For this review, take the finished solid that the model builds, in its own axes (mm). Give positions to 0.01 mm unless a question says otherwise; leave off trailing zeros. Loops run counter-clockwise (first coordinate to the right, second up) from the corner with the lowest first, then second, coordinate; pieces in that order, holes last.
```python
from build123d import *

# Parameters (mm, degrees)
SKETCH1_R           = 3.3782
BOSS_EXTRUDE1_DEPTH = 3.175
FILLET1_R           = 25.4


with BuildPart() as part:
    # Sketch1 → Boss-Extrude1 (new, symmetric)
    with BuildSketch(Plane(origin=(-76.913317281, 0, 0), x_dir=(0, 0, -1), z_dir=(1, 0, 0))):
        with BuildLine():
            Line((535.218804975, 907.961983625), (418.2911251, 916.04381761))
            Line((418.2911251, 916.04381761), (190.115926381, 1052.658490892))
            Line((190.115926381, 1052.658490892), (172.155048622, 1087.522632949))
            ThreePointArc((172.155048622, 1087.522632949), (173.529973777, 1095.130662847), (181.234623159, 1095.771690164))
            Line((181.234623159, 1095.771690164), (418.2911251, 943.327259155))
            Line((418.2911251, 943.327259155), (537.059525989, 923.712003677))
            ThreePointArc((537.059525989, 923.712003677), (543.649965664, 914.959198723), (535.218804975, 907.961983625))
        make_face()
        with Locations((177.8, 1090.430729224)):
            Circle(SKETCH1_R, mode=Mode.SUBTRACT)
        with Locations((434.1661251, 925.56881761)):
            Circle(SKETCH1_R, mode=Mode.SUBTRACT)
        with Locations((535.7661251, 915.880591264)):
            Circle(SKETCH1_R, mode=Mode.SUBTRACT)
    extrude(amount=BOSS_EXTRUDE1_DEPTH, both=True)

    # Fillet1
    fillet1_edges = [part.edges().sort_by_distance(p)[0] for p in [
        (-76.913317281, 916.04381761, -418.2911251),
        (-76.913317281, 1052.658490892, -190.115926381),
        (-76.913317281, 943.327259155, -418.2911251),
    ]]
    fillet(fillet1_edges, radius=FILLET1_R)


solid = part.part
```
Q1. Consider section B-B on x = -78.25. Count the separate pieces of the cut face and the enclosed holes in it, plus the area to 3 significant figures.
Answers:
separate pieces: 1
enclosed holes: 3
area: 10,300 mm2
Q2. Consider section A-A on z = -177.8. Give the boundary of the cut face in (x, y).
Answers:
outline: (-80.09, 1076.57) - (-73.74, 1076.57) - (-73.74, 1087.05) - (-80.09, 1087.05) - close; (-80.09, 1093.81) - (-73.74, 1093.81) - (-73.74, 1096.78) - (-80.09, 1096.78) - close
Q3. Consider section C-C on z = -455. Give the boundary of the cut face in (x, y).
Answers:
outline: (-80.09, 913.51) - (-73.74, 913.51) - (-73.74, 937.26) - (-80.09, 937.26) - close
Q4. Mouldability with a two-part tool opening along Y and no side actions: class faces 1 (the flat face through (-73.738, 982, -345)), 2 (the flat face through (-76.87, 911.74, -480.57)), 3 (the cylindrical face through (-76.958, 1087.133, -177.068)) as +Y half, -Y half, draft (parallel to the pull), parting line (faces both ways), or undercut.
Answers:
face 1: draft
face 2: -Y half
face 3: undercut
Q5. For pin 1 Ø4 at (y, z) = (1090.43, -177.8) entering from -X; pin 2 Ø2 at (x, z) = (-74.5, -285.5) entering from +Y; pin 3 Ø1 at (x, z) = (-75, -311) entering from -Y, all flat-tipped, find the tip position at first contact; note any pin that passes through.
Answers:
pin 1: passes through
pin 2: stops at y = 1029.36
pin 3: stops at y = 979.98
Q6. Consider section D-D on y = 1066.5. Give the boundary of the cut face in (x, z).
Answers:
outline: (-80.09, -226.75) - (-73.74, -226.75) - (-73.74, -182.99) - (-80.09, -182.99) - close
Q7. For probe 1 along Y at (x, z) = (-77, -177.8); probe 2 along Z at (x, y) = (-75, 951); probe 3 along Z at (x, y) = (-79.5, 967), list the stretches that pass through material, from the lowest coordinate up.
Answers:
probe 1: y = 1076.57 to 1087.05, 1093.81 to 1096.78
probe 2: z = -406.36 to -359.91
probe 3: z = -381.48 to -333.18
